Read the model definition and answer for the solid it produces. Units are mm, in the model's axes. Coordinates: 2 decimals unless noted, no trailing zeros. Loops run counter-clockwise (first coordinate to the right, second up) from the corner with the lowest first, then second, coordinate; pieces in that order, holes last. Notation, with made-up numbers: (46.5, 13.5) -> (58.5, 13.5) arc R16 cw to (58.5, 28.5) -> close; hole circle Ø4 at (41, -39). An arc over 180 degrees is marked (long way). Answer as CSV lines item,"result".
```python
from build123d import *

# Parameters (mm, degrees)
F0_W     = 450
F0_H     = 25
F1_DEPTH = 450
F2_SIZE  = 24.99999
F3_SIZE  = 24.99999
F4_SIZE  = 5


# Not quite as in the source:
# - a fillet or chamfer is up to 0.001 mm smaller than in the source, because OpenCascade refuses the exact size


with BuildPart() as f1:
    # F0 (on Front) → F1 (new body)
    with BuildSketch(Plane.XZ):
        with Locations((269.2221287504, -20.1100035338)):
            Rectangle(F0_W, F0_H)
    extrude(amount=F1_DEPTH)

    # F2 (size 25 in the source; OpenCascade refuses exactly that, so slightly less here)
    f2_edges = [f1.edges().sort_by_distance(p)[0] for p in [
        (44.222129, -225, -7.610004),
    ]]
    chamfer(f2_edges, length=F2_SIZE)

    # F3 (size 25 in the source; OpenCascade refuses exactly that, so slightly less here)
    f3_edges = [f1.edges().sort_by_distance(p)[0] for p in [
        (494.222129, -225, -7.610004),
    ]]
    chamfer(f3_edges, length=F3_SIZE)

    # F4
    f4_edges = [f1.edges().sort_by_distance(p)[0] for p in [
        (269.222129, -450, -32.610004),
        (269.222129, 0, -32.610004),
    ]]
    chamfer(f4_edges, length=F4_SIZE)


solid = f1.part
```
Q1. A cutting plane is placed at B-B, the plane z = -20. Write down the section's boundary in (x, y), and give its area (3 significant figures).
Results:
outline,"(56.83, -450) -> (481.61, -450) -> (481.61, 0) -> (56.83, 0) -> close"
area,"191,000 mm²"
Q2. Find the intervals of material crossed by probe 1 along X at (y, z) = (-356, -26.25); probe 2 along X at (y, z) = (-258.5, -22.5); probe 3 along Y at (x, z) = (258, -30.75), in increasing order. Write a range as [from, to].
Results:
probe 1,"x = [50.58, 487.86]"
probe 2,"x = [54.33, 484.11]"
probe 3,"y = [-446.86, -3.14]"
Q3. Given pin 1 Ø1.5 at (y, z) = (-146.5, -15) entering from -X, flat-ended and moving along its own axis, determine where the tip first touches the part or whether it passes through.
Results:
pin 1,"stops at x = 61.08"
